Check sheet for the modelled part. Datum: model origin and axes. Units: mm. Round coordinates to 2 decimals unless told otherwise and drop trailing zeros. Order: outer loops, then holes, each group sorted by start corner. A loop starts at its lowest first (then second) coordinate and runs counter-clockwise, first axis right, second up.
Autodesk Inventor part; units mm, degrees
ref_plane "YZ Plane" through (0, 0, 0) normal (1, 0, 0) x (0, 1, 0)
ref_plane "XZ Plane" through (0, 0, 0) normal (0, 1, 0) x (-1, 0, 0)
ref_plane "XY Plane" through (0, 0, 0) normal (0, 0, 1) x (1, 0, 0)
sketch "Sketch1" plane through (0, 0, 0) normal (0, 0, 1) x (1, 0, 0)
  line L0 (57, -1) -> (1, -1)
  line L1 (1, -1) -> (1, -13)
  arc A0 (-5, -19) -> (1, -13) centre (-5, -13) ccw
  line L2 (-5, -19) -> (-6, -19)
  arc A1 (-6, -19) -> (-10, -23) centre (-6, -23) ccw
  line L3 (-10, -23) -> (-10, -25)
  arc A2 (-10, -25) -> (-6, -29) centre (-6, -25) ccw
  line L4 (-6, -29) -> (-5, -29)
  arc A3 (1, -35) -> (-5, -29) centre (-5, -35) ccw
  line L5 (1, -35) -> (1, -47)
  line L6 (1, -47) -> (57, -47)
  line L7 (57, -47) -> (57, -29)
  line L8 (57, -29) -> (61, -29)
  arc A4 (61, -29) -> (62, -28) centre (61, -28) ccw
  line L9 (62, -28) -> (62, -20)
  arc A5 (62, -20) -> (61, -19) centre (61, -20) ccw
  line L10 (61, -19) -> (57, -19)
  line L11 (57, -19) -> (57, -1)
  point P0 (0, 0)
extrude "Extrusion1" add sketch "Sketch1" along normal blind 2
sketch "Sketch2" plane through (0, 0, 2) normal (0, 0, 1) x (1, 0, 0)
  line L0 (-10, -24) -> (-6, -24) construction
  circle A0 centre (-6, -24) radius 1
  line L1 (-10, -24) -> (-6, -24) construction
  point P0 (0, 0)
  point P1 (-10, -23)
  point P2 (-10, -25)
  dimension "d14" = 2
  dimension "d20" = 4
extrude "Extrusion2" cut sketch "Sketch2" against normal blind 5
thread "Thread1"
properties part number "Battery holder lid"
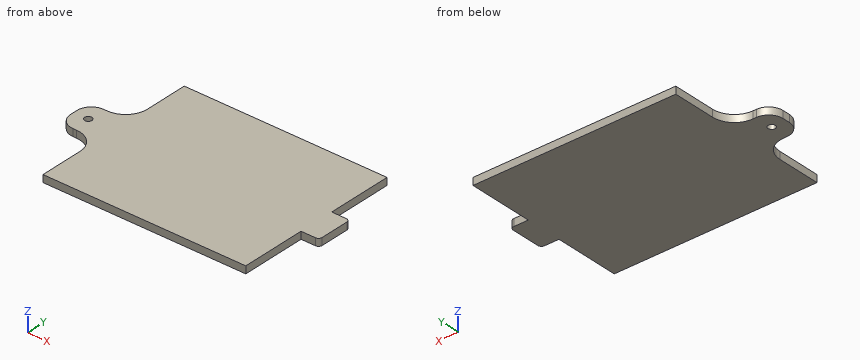
Item 1: Sectioned sample at C-C (y = -10.5). Record the cut outline in (x, z), and give its area (3 significant figures).
Answer:
outline: (1, 0) - (57, 0) - (57, 2) - (1, 2) - close
area: 112 mm2
Item 2: Sectioned sample at B-B (z = 1). Record the cut outline in (x, y).
Answer:
outline: (-10, -25) arc R4 ccw to (-6, -29) - (-5, -29) arc R6 cw to (1, -35) - (1, -47) - (57, -47) - (57, -29) - (61, -29) arc R1 ccw to (62, -28) - (62, -20) arc R1 ccw to (61, -19) - (57, -19) - (57, -1) - (1, -1) - (1, -13) arc R6 cw to (-5, -19) - (-6, -19) arc R4 ccw to (-10, -23) - close; hole circle Ø2 at (-6, -24)
Item 3: Sectioned sample at A-A (y = -24). Record the cut outline in (x, z).
Answer:
outline: (-10, 0) - (-7, 0) - (-7, 2) - (-10, 2) - close; (-5, 0) - (62, 0) - (62, 2) - (-5, 2) - close
Item 4: Scan lines: line 1 along Y through (x, z) = (-6, 0.5); line 2 along X through (y, z) = (-12, 1.7); line 3 along X through (y, z) = (-23.5, 0.15). Record each from-to range of solid material in increasing order.
Answer:
line 1: y = -29 to -25, -23 to -19
line 2: x = 1 to 57
line 3: x = -10 to -6.87, -5.13 to 62
Item 5: Go/stop test with flat-tipped pins: P1, Ø1, axis at y = -36, z = 0.5, coming from the +X side; P2, Ø3, axis at x = -6, y = -24, coming from the -Z side; P3, Ø0.8, axis at x = -5.5, z = 0.5, coming from the +Y side; P4, Ø0.8, axis at x = -5.5, z = 1, coming from the -Y side. Record where each tip stops, or that it passes through.
Answer:
P1: stops at x = 57
P2: stops at z = 0
P3: stops at y = -19
P4: stops at y = -29
Item 6: Sectioned sample at D-D (y = -33.5). Record the cut outline in (x, z), and give its area (3 significant figures).
Answer:
outline: (0.81, 0) - (57, 0) - (57, 2) - (0.81, 2) - close
area: 112 mm2
